Source: CAD feature listing. Evaluate the final solid. Frame: model axes, mm. A direction names the side the tool comes from. Give positions to 0.01 mm unless a question says otherwise; leave off trailing zeros. Loops run counter-clockwise (first coordinate to the right, second up) from the corner with the lowest first, then second, coordinate; pieces in that order, holes last. Notation, with made-up numbers: (81, -3.5) - (115, -3.5) arc R28 cw to (115, 24.5) - close; hole circle Ø4 at (33, -19.75). An arc over 180 degrees is marked (long way). Put each result on its own line as item: value.
```python
from build123d import *

# Parameters (mm, degrees)
SKETCH2_R               = 180
BOSS_EXTRUDE1_DEPTH     = 9
SKETCH3_W               = 5
SKETCH3_H               = 185
BOSS_EXTRUDE2_DEPTH     = 310
SKETCH7_R               = 4.5
CUT_EXTRUDE2_DEPTH      = 181
CUT_EXTRUDE2_DEPTH_BACK = 181


with BuildPart() as part:
    # Sketch2 → Boss-Extrude1 (new body)
    with BuildSketch(Plane(origin=(0, 0, 0), x_dir=(1, 0, 0), z_dir=(0, 1, 0))):
        Circle(SKETCH2_R)
    extrude(amount=-BOSS_EXTRUDE1_DEPTH)

    # Sketch3 → Boss-Extrude2 (add)
    with BuildSketch(Plane(origin=(0, 0, 0), x_dir=(1, 0, 0), z_dir=(0, 1, 0))):
        with Locations((-100, 0)):
            Rectangle(SKETCH3_W, SKETCH3_H)
        with Locations((100, 0)):
            Rectangle(SKETCH3_W, SKETCH3_H)
    extrude(amount=BOSS_EXTRUDE2_DEPTH)

    # Sketch7 → Cut-Extrude2 (cut, two sides)
    with BuildSketch(Plane(origin=(0, 0, 0), x_dir=(0, 0, -1), z_dir=(1, 0, 0))) as cut_extrude2_sk:
        with Locations((0, 230)):
            Circle(SKETCH7_R)
    extrude(amount=CUT_EXTRUDE2_DEPTH, mode=Mode.SUBTRACT)
    extrude(cut_extrude2_sk.sketch, amount=-CUT_EXTRUDE2_DEPTH_BACK, mode=Mode.SUBTRACT)


solid = part.part
```
1) Material intervals for line 1 along Y through (x, z) = (-100.05, 0); line 2 along Z through (x, y) = (100, 230); line 3 along X through (y, z) = (104, -51.5), sorted ascending. Write a range as [from, to].
Check result:
line 1: [-9, 225.5], [234.5, 310]
line 2: [-92.5, -4.5], [4.5, 92.5]
line 3: [-102.5, -97.5], [97.5, 102.5]
2) Mould query, pull axis X, two halves, no side actions, for faces 3 (the flat face through (-102.5, 153, 1)), 4 (the flat face through (-97.5, 153, 1)), 5 (the flat face through (-3, -9, -3)), 6 (the flat face through (97.5, 153, 1)). Classes: pulls with the +X half, pulls with the -X half, needs draft (parallel to the pull), parting line crosses it, or undercut.
Check result:
face 3: pulls with the -X half
face 4: undercut
face 5: needs draft
face 6: undercut
3) Access query for faces 1 (the flat face through (102.5, 153, 1)), 2 (the cylindrical face through (83.06, -4.44, 159.69)). Directions: +Z, -Z, +X, -X, +Y, -Y. A direction counts if a zero-diameter tool reaches every point of the face in a straight line with its end or side. Return the directions, or none.
Check result:
face 1: +Z, -Z, +X, +Y
face 2: +Y, -Y
4) Section query B-B, the plane z = -44. Output: boundary loops of the cut face in (x, y).
Check result:
outline: (-174.54, -9) - (174.54, -9) - (174.54, 0) - (102.5, 0) - (102.5, 310) - (97.5, 310) - (97.5, 0) - (-97.5, 0) - (-97.5, 310) - (-102.5, 310) - (-102.5, 0) - (-174.54, 0) - close
5) Pin query (flat end, axial travel): P1, Ø1.5, axis at x = 99.5, y = 228, coming from the -Z side; P2, Ø6, axis at y = 257.5, z = -76, coming from the +X side; P3, Ø1.5, axis at x = 131.5, z = 57.5, coming from the +Y side; P4, Ø7, axis at y = 230, z = 0, coming from the +X side. Return the tip coordinate at first contact, or that it passes through.
Check result:
P1: z = -92.5
P2: x = 102.5
P3: y = 0
P4: through
6) Section query A-A, the plane y = 71.5. Output: boundary loops of the cut face in (x, z), plus the area to 3 significant figures.
Check result:
outline: (-102.5, -92.5) - (-97.5, -92.5) - (-97.5, 92.5) - (-102.5, 92.5) - close; (97.5, -92.5) - (102.5, -92.5) - (102.5, 92.5) - (97.5, 92.5) - close
area: 1,850 mm²
7) Section query D-D, the plane x = 81.5. Output: boundary loops of the cut face in (y, z).
Check result:
outline: (-9, -160.49) - (0, -160.49) - (0, 160.49) - (-9, 160.49) - close
8) Section query C-C, the plane x = 0. Output: boundary loops of the cut face in (y, z), plus the area to 3 significant figures.
Check result:
outline: (-9, -180) - (0, -180) - (0, 180) - (-9, 180) - close
area: 3,240 mm²
